Solid Edge part; units mm, degrees
sketch "Sketch1" plane through (-58.5972, 0, 0) normal (1, 0, 0) x (0, 1, 0)
  line L0 (55.0553, 59.6775) -> (52.5553, 59.6775)
  line L1 (52.5553, 59.6775) -> (55.38, 66.2556)
  line L2 (65.5553, 59.6775) -> (62.7304, 66.2556)
  line L3 (65.5553, 59.6775) -> (63.0553, 59.6775)
  line L4 (63.0553, 56.6775) -> (63.0553, 59.6775)
  line L5 (55.0553, 56.6775) -> (63.0553, 56.6775)
  line L6 (55.0553, 59.6775) -> (55.0553, 56.6775)
  arc A0 (55.38, 66.2556) -> (62.7304, 66.2556) centre (59.0552, 64.6774) cw
  circle A1 centre (59.0552, 64.6774) radius 0.8
extrude "Protrusion1" add sketch "Sketch1" along normal blind 4
Can you work these out from the model? Positions are in its coordinate system, mm. A direction names the side the tool comes from. Coordinates: 2 decimals unless noted, no trailing zeros. Write each loop counter-clockwise with the first axis right and the second up, starting at its lowest first coordinate (ties: lowest second). Pieces come first, ordered by that corner, then holes. Notation, with made-up numbers: (45, 24) -> (60, 24) arc R21 cw to (60, 46) -> close; hole circle Ø7 at (19.25, 38). An arc over 180 degrees is marked (long way). Write each question's results on one line, items separated by ' | '. Start each with the question number.
Q1. We'd pull the mould along Z, two halves only. Please class faces 4 (the face through (-54.597, 59, 63)), 5 (the face through (-56.63, 58.88, 65.46)), 6 (the face through (-56.625, 64.163, 62.921)): +Z half, -Z half, draft (parallel to the pull), parting line (faces both ways), or undercut.
Q2. On a 3-axis mill with a long thin cutter (end or side, diameter ignored), from which of +Z, -Z, +X, -X, +Y, -Y can I reach the whole of each face in a straight line? I mean faces 1 (the face through (-57, 54, 59.678)), 2 (the face through (-57, 63.055, 58)), 3 (the face through (-56.625, 53.948, 62.921)). Say none if no direction works.
Q3. If I drill on probe 1 along Z at (x, y) = (-56, 59); probe 2 along Z at (x, y) = (-55.65, 63.75); probe 3 along Y at (x, z) = (-56.1, 58), over which ranges is the centre line in solid material (lowest first)?
Q4. Imagine slicing it at B-B (z = 65). Write out the boundary of the cut face in (x, y).
Q5. I'm going to push flat-ended pins straight in: pin 1 (1.2 mm diameter, centred on x = -57.5, y = 53.5, fed in from -Z); pin 2 (1.5 mm diameter, centred on x = -56, z = 61.5, fed in from -Y); pin 3 (1.5 mm diameter, centred on x = -57, z = 59, fed in from +Y); pin 4 (1.5 mm diameter, centred on x = -57.5, z = 58, fed in from -Y). Where does each tip first touch, or does it pass through?
Q6. Imagine slicing it at A-A (y = 59.5). Write out the boundary of the cut face in (x, z).
Q7. Imagine slicing it at C-C (x = -56.95). Write out the boundary of the cut face in (y, z).
Q8. Imagine slicing it at D-D (z = 57.75). Write out the boundary of the cut face in (x, y), then the cut area to 3 significant figures.
Taken from the geometry:
1) face 4: draft | face 5: undercut | face 6: +Z half
2) face 1: -Z, +X, -X, -Y | face 2: -Z, +X, -X, +Y | face 3: +Z, +X, -X, -Y
3) probe 1: z = 56.68 to 63.88, 65.48 to 68.68 | probe 2: z = 59.68 to 63.88 | probe 3: y = 55.06 to 63.06
4) outline: (-58.6, 54.84) -> (-54.6, 54.84) -> (-54.6, 58.32) -> (-58.6, 58.32) -> close; (-58.6, 59.79) -> (-54.6, 59.79) -> (-54.6, 63.27) -> (-58.6, 63.27) -> close
5) pin 1: stops at z = 59.68 | pin 2: stops at y = 53.02 | pin 3: stops at y = 65.56 | pin 4: stops at y = 55.06
6) outline: (-58.6, 56.68) -> (-54.6, 56.68) -> (-54.6, 64.01) -> (-58.6, 64.01) -> close; (-58.6, 65.34) -> (-54.6, 65.34) -> (-54.6, 68.65) -> (-58.6, 68.65) -> close
7) outline: (52.56, 59.68) -> (55.06, 59.68) -> (55.06, 56.68) -> (63.06, 56.68) -> (63.06, 59.68) -> (65.56, 59.68) -> (62.73, 66.26) arc R4 ccw to (55.38, 66.26) -> close; hole circle Ø1.6 at (59.06, 64.68)
8) outline: (-58.6, 55.06) -> (-54.6, 55.06) -> (-54.6, 63.06) -> (-58.6, 63.06) -> close | area: 32.0 mm^2
